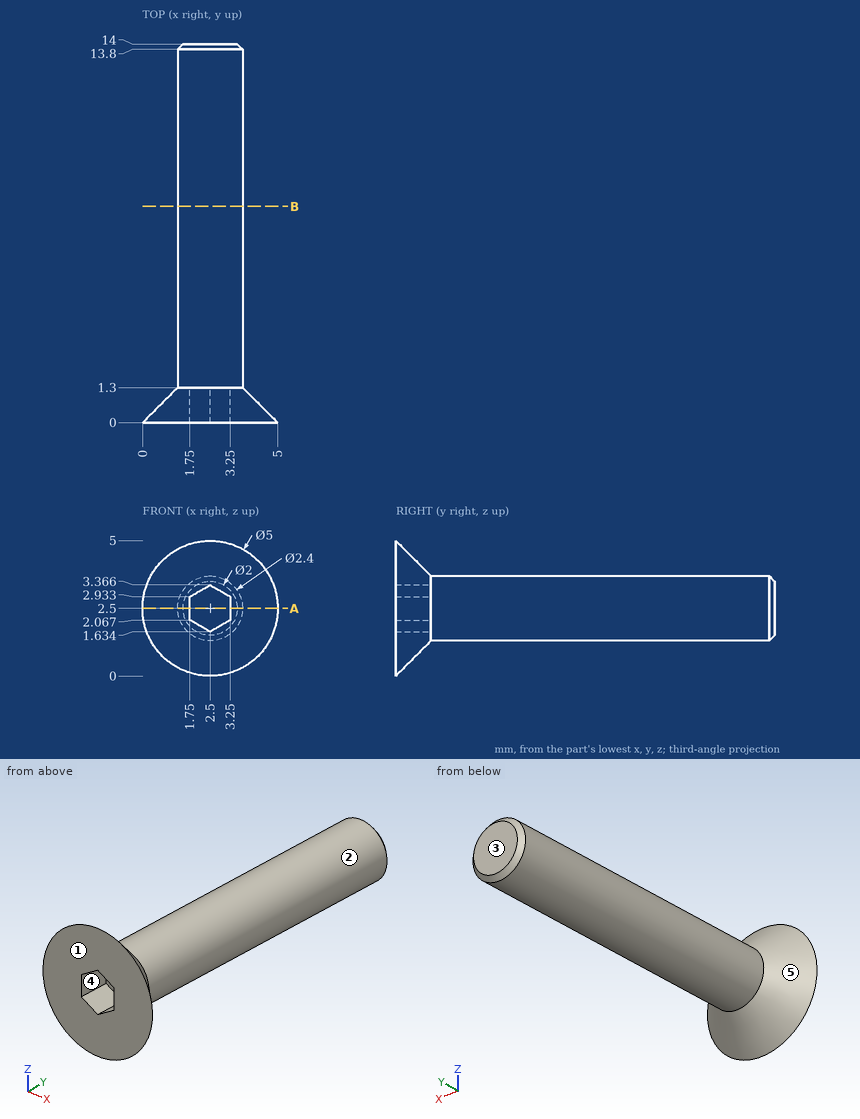
Input: dimensioned drawing with shaded views. Units: mm. Origin: part minimum x, y, z. A direction names the side the tool comes from. Give positions to 0.01 mm unless a question says otherwise; leave off trailing zeros. Write each loop counter-clockwise with the first axis right and the second up, starting at its lowest first coordinate (ties: lowest second). Pieces come first, ordered by that corner, then holes. Notation, with made-up numbers: (-27.5, 8.25) -> (-8.5, 8.25) arc R20 ccw to (-8.5, 13.25) -> close; hole circle Ø11 at (11.5, -18.5). An arc over 180 degrees is marked (long way). Return JSON: item names as keys, results as strings. Group by question number.
1. Access query for the marked faces 1 and 2. Directions: +Z, -Z, +X, -X, +Y, -Y. A direction counts if a zero-diameter tool reaches every point of the face in a straight line with its end or side. Return the directions, or none.
2. Material intervals for line 1 (Y direction, x = 2.2, z = 2.8); line 2 (Y direction, x = 1.35, z = 1.65); line 3 (X direction, y = 0.5, z = 2.9), sorted ascending. Write a range as from..to.
3. Section B-B, the plane y = 8. Output: boundary loops of the cut face in (x, z), then the cut area to 3 significant figures.
4. Section A-A, the plane z = 2.5. Output: boundary loops of the cut face in (x, y), then the cut area to 3 significant figures.
5. Mould query, pull axis Z, two halves, no side actions, for the marked faces 3, 4 and 5. Classes: +Z half, -Z half, draft (parallel to the pull), parting line (faces both ways), or undercut.
6. Pin query (flat end, axial travel): pin 1 Ø0.7 at (y, z) = (0.5, 2.5) entering from +X; pin 2 Ø1.5 at (y, z) = (6.5, 1) entering from -X. Return the tip coordinate at first contact, or that it passes through.
Determined:
{
 "1": {"face 1": "+Z, -Z, +X, -X, -Y", "face 2": "+Y"},
 "2": {"line 1": "y = 1.3..14", "line 2": "y = 0..1.07", "line 3": "x = 0.54..1.75, 3.25..4.46"},
 "3": {"outline": "circle Ø2.4 at (2.5, 2.5)", "area": "4.52 mm2"},
 "4": {"outline": "(0, 0) -> (1.75, 0) -> (1.75, 1.3) -> (3.25, 1.3) -> (3.25, 0) -> (5, 0) -> (3.7, 1.3) -> (3.7, 13.8) -> (3.5, 14) -> (1.5, 14) -> (1.3, 13.8) -> (1.3, 1.3) -> close", "area": "33.3 mm2"},
 "5": {"face 3": "draft", "face 4": "undercut", "face 5": "parting line"},
 "6": {"pin 1": "stops at x = 4.85", "pin 2": "stops at x = 1.56"}
}
